Verification items for this drawing (mm, ordinates from the low corner). A direction names the side the tool comes from. Coordinates: 2 decimals unless noted, no trailing zeros. Loops run counter-clockwise (first coordinate to the right, second up) from the corner with the lowest first, then second, coordinate; pieces in that order, holes last. Notation, with made-up numbers: M 21.25,36.25 L 59.25,36.25 A11 ccw 59.25,42.25 Z; hole C 34.25,11 d9. An arc over 180 degrees is marked long. Write each question's results on one line, items separated by ' | '. Start each with the question number.
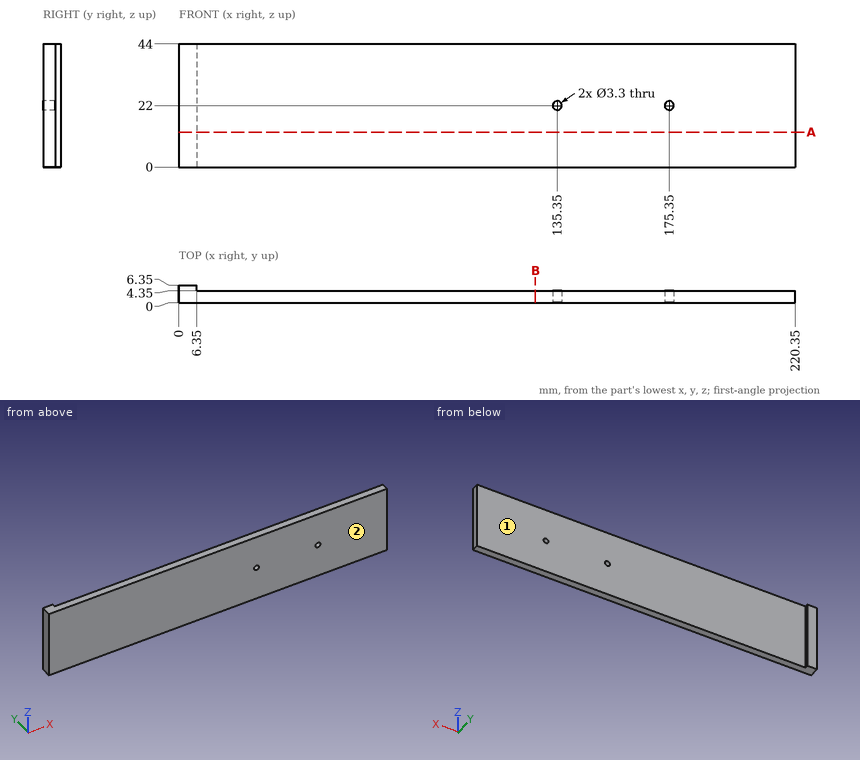
Item 1: Section check B-B (x = 127.5). Record the cut outline in (y, z), plus the area to 3 significant figures.
Item 2: Thickness scan on line 1 (X direction, y = 2.6, z = 22); line 2 (Z direction, x = 135.35, y = 1.6); line 3 (X direction, y = 5, z = 18.5). Record the ranges inside material, lowest first.
Item 3: Depth check by flat-ended pin: P1, Ø1, axis at x = 42, z = 25, coming from the +Y side; P2, Ø1.5, axis at y = 5.5, z = 19, coming from the +X side; P3, Ø2.5, axis at x = 175.35, z = 22, coming from the -Y side. Enter the tip coordinate at first touch or a pass-through.
Item 4: Tool access check on the marked faces 1 and 2. Record the directions out of +Z, -Z, +X, -X, +Y, -Y that give a thin tool (end or side, any length) a straight path to the whole face; none if there is none.
Item 5: Section check A-A (z = 12.5). Record the cut outline in (x, y), plus the area to 3 significant figures.
Computed values:
1) outline: M 0,0 L 4.35,0 L 4.35,44 L 0,44 Z | area: 191 mm²
2) line 1: x = 0 to 133.7, 137 to 173.7, 177 to 220.35 | line 2: z = 0 to 20.35, 23.65 to 44 | line 3: x = 0 to 6.35
3) P1: stops at y = 4.35 | P2: stops at x = 6.35 | P3: passes through
4) face 1: +Z, -Z, +X, +Y | face 2: +Z, -Z, +X, -X, -Y
5) outline: M 0,0 L 220.35,0 L 220.35,4.35 L 6.35,4.35 L 6.35,6.35 L 0,6.35 Z | area: 971 mm²
